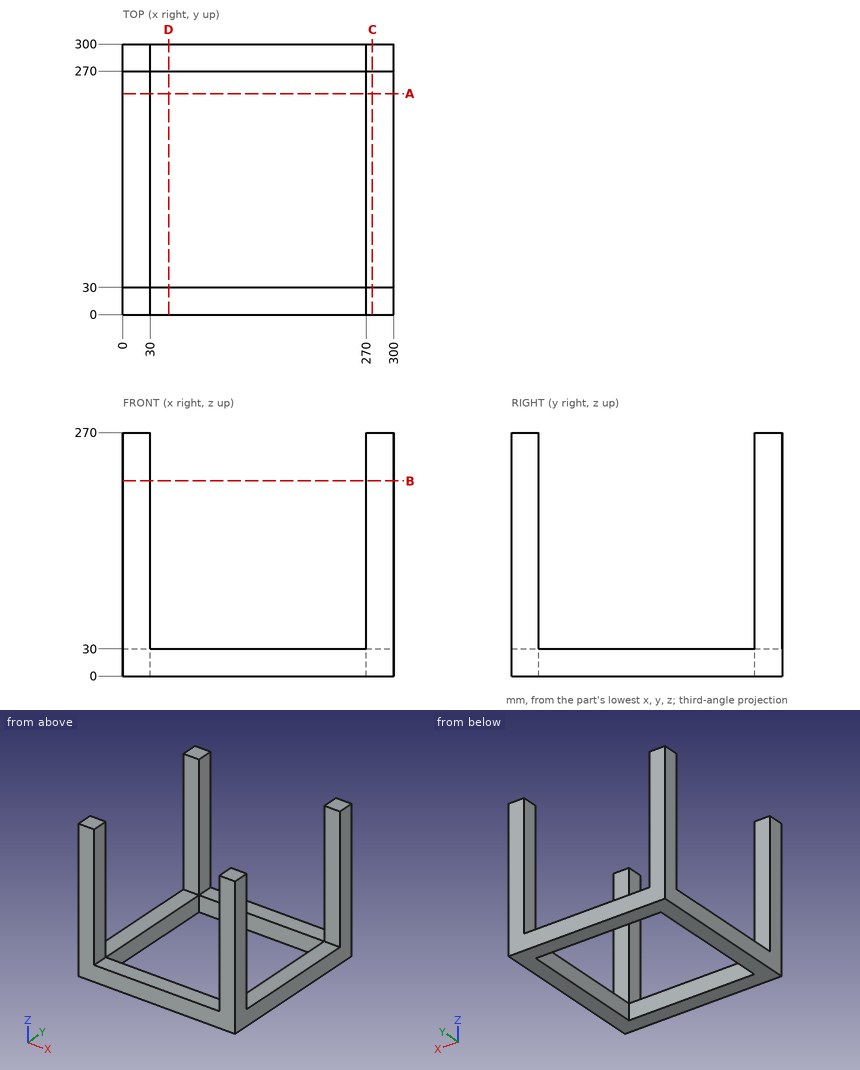
Verification items for this drawing (mm, ordinates from the low corner). Round coordinates to 2 decimals unless told otherwise and drop trailing zeros. Loops run counter-clockwise (first coordinate to the right, second up) from the corner with the lowest first, then second, coordinate; pieces in that order, holes last. Notation, with made-up numbers: (-30, 38) -> (-24, 38) arc R15 cw to (-24, 60) -> close; hole circle Ø1 at (51.25, 50.25). An arc over 180 degrees is marked (long way). Answer in a Markdown table with one row per item.
Q1. Go/stop test with flat-tipped pins: P1, Ø9, axis at x = 13.5, y = 144, coming from the +Z side; P2, Ø15, axis at y = 9, z = 120, coming from the -X side. Record where each tip stops, or that it passes through.
Data:
| item | result |
|---|---|
| P1 | stops at z = 30 |
| P2 | stops at x = 0 |
Q2. Sectioned sample at A-A on y = 245. Enter the section's corners in (x, z), then the cut area to 3 significant figures.
Data:
| item | result |
|---|---|
| outline | (0, 0) -> (30, 0) -> (30, 30) -> (0, 30) -> close; (270, 0) -> (300, 0) -> (300, 30) -> (270, 30) -> close |
| area | 1,800 mm^2 |
Q3. Sectioned sample at C-C on x = 276.5. Enter the section's corners in (y, z).
Data:
| item | result |
|---|---|
| outline | (0, 0) -> (300, 0) -> (300, 270) -> (270, 270) -> (270, 30) -> (30, 30) -> (30, 270) -> (0, 270) -> close |
Q4. Thickness scan on L1, parallel to Y at x = 26.5, z = 159; L2, parallel to Z at x = 140, y = 285.5. Record the ranges inside material, lowest first.
Data:
| item | result |
|---|---|
| L1 | y = 0 to 30, 270 to 300 |
| L2 | z = 0 to 30 |
Q5. Sectioned sample at B-B on z = 216.5. Enter the section's corners in (x, y), then the cut area to 3 significant figures.
Data:
| item | result |
|---|---|
| outline | (0, 0) -> (30, 0) -> (30, 30) -> (0, 30) -> close; (0, 270) -> (30, 270) -> (30, 300) -> (0, 300) -> close; (270, 0) -> (300, 0) -> (300, 30) -> (270, 30) -> close; (270, 270) -> (300, 270) -> (300, 300) -> (270, 300) -> close |
| area | 3,600 mm^2 |
